Read the model definition and answer for the solid it produces. Units are mm, in the model's axes. A direction names the side the tool comes from. Round coordinates to 2 decimals unless told otherwise and drop trailing zeros. Order: outer loops, then holes, each group sorted by start corner. A loop starts at its lowest first (then second) coordinate and runs counter-clockwise, first axis right, second up. Notation, with made-up numbers: (86.25, -15) - (94.25, -15) arc R26 cw to (94.25, 19) - close; hole circle Ø4 at (26.5, 43). An arc over 180 degrees is marked (long way). Answer as a JSON object with one key per item and string values. Group by question number.
Q1. A cutting plane is placed at A-A on z = -4. Determine the outline of the cut face in (x, y).
Q2. A cutting plane is placed at C-C on z = 0. Determine the outline of the cut face in (x, y) (3 decimals), and give its area (3 significant figures).
Q3. Consider line 1 (Z direction, x = 4.5, y = 3.5); line 2 (Y direction, x = 0, z = -2.5); line 3 (X direction, y = 0.25, z = -5.25). Determine where each line is inside the solid, lowest interval first.
Q4. The mould has two halves that part along Y. Classify faces 3 (the cylindrical face through (-0.228, 0.975, -4.5)), 4 (the flat face through (0, 0, -2)), 5 (the flat face through (0, 4, -2)), 6 (the cylindrical face through (6.25, 1.97, 0.04)): pulls with the +Y half, pulls with the -Y half, needs draft (parallel to the pull), parting line crosses it, or undercut.
Q5. A tool of negligible diameter and unlimited length cuts with its end or side. For faces 1 (the flat face through (-1, 1, -1.425)), 2 (the cylindrical face through (-6.25, 1.97, -0.04)), from which of +Z, -Z, +X, -X, +Y, -Y can it reach the whole face along a straight path? Write none if from no direction.
Q6. A cutting plane is placed at D-D on y = 3.65. Determine the outline of the cut face in (x, z) (3 decimals), and give its area (3 significant figures).
Q7. A cutting plane is placed at B-B on x = 0. Determine the outline of the cut face in (y, z) (3 decimals), and give its area (3 significant figures).
Q8. Given pin 1 Ø2 at (x, z) = (4.49, 4.49) entering from +Y; pin 2 Ø1.3 at (x, y) = (0, 2) entering from -Z; pin 3 Ø1 at (y, z) = (2, -0.5) entering from +X, each flat-ended and moving along its own axis, determine where each tip first touches the part or whether it passes through.
```python
from build123d import *

# Parameters (mm, degrees)
SKETCH1_R                 = 0.85
BASE_SHAPE_DEPTH          = 4
M2_5_GRUB_SCREW_CUT_REACH = 16.98
SKETCH3_R                 = 1.05


with BuildPart() as part:
    # Sketch1 → Base shape (new body)
    with BuildSketch(Plane(origin=(0, 0, 0), x_dir=(1, 0, 0), z_dir=(0, 1, 0))):
        with BuildLine():
            Line((4.490128061, 7.490128061), (-4.490128061, 7.490128061))
            ThreePointArc((-4.490128061, 7.490128061), (-7.099636787, 5.970149752), (-7.064881074, 2.950437533))
            ThreePointArc((-7.064881074, 2.950437533), (-6.25, 0), (-7.064881074, -2.950437533))
            ThreePointArc((-7.064881074, -2.950437533), (-7.099636787, -5.970149752), (-4.490128061, -7.490128061))
            Line((-4.490128061, -7.490128061), (4.490128061, -7.490128061))
            ThreePointArc((4.490128061, -7.490128061), (7.099636787, -5.970149752), (7.064881074, -2.950437533))
            ThreePointArc((7.064881074, -2.950437533), (6.25, 0), (7.064881074, 2.950437533))
            ThreePointArc((7.064881074, 2.950437533), (7.099636787, 5.970149752), (4.490128061, 7.490128061))
        make_face()
        with BuildLine():
            Line((-1.438749457, 1.425), (1.438749457, 1.425))
            ThreePointArc((1.438749457, 1.425), (1.859326776, 1.195397336), (1.893641402, 0.717458876))
            ThreePointArc((1.893641402, 0.717458876), (0, -2.025), (-1.893641402, 0.717458876))
            ThreePointArc((-1.893641402, 0.717458876), (-1.859326776, 1.195397336), (-1.438749457, 1.425))
        make_face(mode=Mode.SUBTRACT)
        with Locations((-4.490128061, 4.490128061)):
            Circle(SKETCH1_R, mode=Mode.SUBTRACT)
        with Locations((4.490128061, 4.490128061)):
            Circle(SKETCH1_R, mode=Mode.SUBTRACT)
        with Locations((-4.490128061, -4.490128061)):
            Circle(SKETCH1_R, mode=Mode.SUBTRACT)
        with Locations((4.490128061, -4.490128061)):
            Circle(SKETCH1_R, mode=Mode.SUBTRACT)
    extrude(amount=BASE_SHAPE_DEPTH)

    # Sketch3 → M2.5 Grub screw cut (cut, up to next)
    with BuildSketch(Plane.XY.offset(-7.490128061), mode=Mode.PRIVATE) as m2_5_grub_screw_cut_sk1:
        with Locations((0, 2)):
            Circle(SKETCH3_R)
    m2_5_grub_screw_cut_tool1 = extrude(m2_5_grub_screw_cut_sk1.sketch, amount=M2_5_GRUB_SCREW_CUT_REACH, mode=Mode.PRIVATE) & part.part
    add(m2_5_grub_screw_cut_tool1.solids().sort_by_distance((0, 2, -7.490128))[0], mode=Mode.SUBTRACT)


solid = part.part
```
Result set:
{
 "1": {"outline": "(-7.45, 0) - (-5.18, 0) - (-5.18, 4) - (-7.45, 4) - close; (-3.8, 0) - (3.8, 0) - (3.8, 4) - (-3.8, 4) - close; (5.18, 0) - (7.45, 0) - (7.45, 4) - (5.18, 4) - close; hole circle Ø2.1 at (0, 2)"},
 "2": {"outline": "(-6.25, 0) - (-2.025, 0) - (-2.025, 4) - (-6.25, 4) - close; (2.025, 0) - (6.25, 0) - (6.25, 4) - (2.025, 4) - close", "area": "33.8 mm²"},
 "3": {"line 1": "z = -7.49 to -5.34, -3.64 to 3.64, 5.34 to 7.49", "line 2": "y = 0 to 0.95, 3.05 to 4", "line 3": "x = -7.39 to -4.87, -4.11 to 4.11, 4.87 to 7.39"},
 "4": {"face 3": "undercut", "face 4": "pulls with the -Y half", "face 5": "pulls with the +Y half", "face 6": "needs draft"},
 "5": {"face 1": "+Y, -Y", "face 2": "-X, +Y, -Y"},
 "6": {"outline": "(-7.065, -2.95) arc R3 ccw to (-4.49, -7.49) - (4.49, -7.49) arc R3 ccw to (7.065, -2.95) arc R5.749 cw to (7.065, 2.95) arc R3 ccw to (4.49, 7.49) - (-4.49, 7.49) arc R3 ccw to (-7.065, 2.95) arc R5.749 cw to start; hole circle Ø1.7 at (-4.49, -4.49); hole circle Ø1.7 at (-4.49, 4.49); hole (-1.894, -0.717) arc R0.5 ccw to (-1.439, -1.425) - (1.439, -1.425) arc R0.5 ccw to (1.894, -0.717) arc R2.025 ccw (long way) to start; hole circle Ø1.7 at (4.49, -4.49); hole circle Ø1.7 at (4.49, 4.49)", "area": "183 mm²"},
 "7": {"outline": "(0, -7.49) - (0.95, -7.49) - (0.95, -1.425) - (0, -1.425) - close; (0, 2.025) - (4, 2.025) - (4, 7.49) - (0, 7.49) - close; (3.05, -7.49) - (4, -7.49) - (4, -1.425) - (3.05, -1.425) - close", "area": "33.4 mm²"},
 "8": {"pin 1": "stops at y = 4", "pin 2": "stops at z = 1.92", "pin 3": "stops at x = 6.34"}
}
